Autodesk Inventor part; units mm, degrees
ref_plane "YZ Plane" through (0, 0, 0) normal (1, 0, 0) x (0, 1, 0)
ref_plane "XZ Plane" through (0, 0, 0) normal (0, 1, 0) x (-1, 0, 0)
ref_plane "XY Plane" through (0, 0, 0) normal (0, 0, 1) x (1, 0, 0)
sketch "Sketch1" plane through (0, 0, 0) normal (0, 0, 1) x (1, 0, 0)
  circle A0 centre (0, 0) radius 44.45
  line L0 (-44.45, 44.45) -> (44.45, 44.45)
  line L1 (44.45, 44.45) -> (44.45, -44.45)
  line L2 (44.45, -44.45) -> (-44.45, -44.45)
  line L3 (-44.45, -44.45) -> (-44.45, 44.45)
  dimension "d0" = 88.9
  dimension "d1" = 88.9
  dimension "d2" = 88.9
  dimension "d3" = 44.45
  dimension "d4" = 44.45
extrude "Extrusion1" add sketch "Sketch1" along normal blind 6.35
sketch "Sketch2" plane through (0, 0, 6.35) normal (0, 0, 1) x (1, 0, 0)
  circle A0 centre (0, 0) radius 46.0375
  circle A1 centre (0, 0) radius 44.45
  circle A2 centre (0, 0) radius 39.6875
  dimension "d8" = 1.5875
  dimension "d46" = 88.9
  dimension "d82" = 79.375
extrude "Extrusion2" add sketch "Sketch2" along normal blind 25.4 contours A1
sketch "Sketch3" plane through (0, 0, 6.35) normal (0, 0, 1) x (1, 0, 0)
  circle A0 centre (0, 0) radius 14.2875
  dimension "d11" = 28.575
extrude "Extrusion3" cut sketch "Sketch3" against normal blind 38.1
sketch "Sketch4" plane through (0, 0, 6.35) normal (0, 0, 1) x (1, 0, 0)
  circle A0 centre (0, 0) radius 14.2875
  circle A1 centre (0, 0) radius 19.05
  dimension "d14" = 38.1
extrude "Extrusion4" add sketch "Sketch4" along normal blind 25.4
sketch "Sketch7" plane through (0, 0, 6.35) normal (0, 0, 1) x (1, 0, 0)
  line L0 (44.45, 44.45) -> (0, 44.45)
  line L1 (-44.45, 44.45) -> (-44.45, 0)
  line L2 (-44.45, -44.45) -> (0, -44.45)
  line L3 (44.45, -44.45) -> (44.45, 0)
  line L4 (44.45, -44.45) -> (44.45, 44.45)
  line L5 (-44.45, 0) -> (-44.45, -44.45)
  line L6 (-44.45, -44.45) -> (0, -44.45)
  line L7 (44.45, -44.45) -> (-44.45, -44.45)
  line L8 (0, -44.45) -> (44.45, -44.45)
  line L9 (44.45, -44.45) -> (44.45, 0)
  arc A0 (-44.45, 0) -> (0, -44.45) centre (0, 0) ccw
  arc A1 (0, -44.45) -> (44.45, 0) centre (0, 0) ccw
  arc A2 (44.45, 0) -> (0, 44.45) centre (0, 0) ccw
  line L10 (44.45, 0) -> (44.45, 44.45)
  arc A3 (0, 44.45) -> (-44.45, 0) centre (0, 0) ccw
  line L11 (0, 44.45) -> (-44.45, 44.45)
  arc A4 (-44.45, 0) -> (0, -44.45) centre (0, 0) ccw
  line L12 (-44.45, 0) -> (-44.45, -44.45)
  arc A5 (0, -44.45) -> (44.45, 0) centre (0, 0) ccw
  line L13 (0, -44.45) -> (44.45, -44.45)
  point P0 (-44.4261, -1.4578)
  point P1 (44.4261, -1.4578)
extrude "Extrusion7" [suppressed]
sketch "Sketch8" plane through (0, 0, 0) normal (0, 1, 0) x (-1, 0, 0)
  line L0 (44.45, 6.35) -> (44.45, 31.75)
  arc A0 (44.45, 28.2575) -> (44.45, 22.5425) centre (45.974, 25.4) ccw
  line L1 (44.45, 31.75) -> (-44.45, 31.75)
  line L2 (0, -7.62) -> (0, 45.72)
  arc A1 (44.2147, 22.6811) -> (44.45, 28.2575) centre (45.974, 25.4) ccw
  point P0 (0, 0)
  dimension "d28" = 3.2385
  dimension "d31" = 19.05
  dimension "d45" = 1.7145
revolve "Revolution1" cut sketch "Sketch8" angle 360 about axis through (0, 0, -10) along (0, 0, 1) contours A0 L0
sketch "Sketch11" plane through (0, 0, 0) normal (0, 1, 0) x (-1, 0, 0)
  line L0 (-19.05, 6.35) -> (-19.05, 31.75)
  line L1 (-19.05, 38.1) -> (-26.605, 25.4)
  line L2 (-26.605, 25.4) -> (-23.8011, 25.4)
  line L3 (44.45, 28.2575) -> (-44.45, 28.2575)
  line L4 (-23.8011, 25.4) -> (-17.684, 35.6829)
  point P0 (0, 0)
  dimension "d43" = 25.4
  dimension "d44" = 12.7
sketch "Sketch12" plane through (-44.45, 44.45, 0) normal (0, 1, 0) x (1, 0, 0)
  line L0 (0, 0) -> (88.9, 0)
  line L1 (0, 0) -> (0, -6.35)
  line L2 (44.45, -6.35) -> (0, -6.35)
  line L3 (88.9, 0) -> (88.9, -6.35)
  line L4 (88.9, -6.35) -> (44.45, -6.35)
  point P0 (44.45, 0)
sketch "Sketch13" plane through (0, 0, 0) normal (0, 0, -1) x (-1, 0, 0)
  circle A0 centre (0, 0) radius 44.45
  arc A1 (-44.45, 0) -> (0, -44.45) centre (0, 0) ccw
  line L0 (-7.4513, 43.821) -> (0.0223, 44.45)
  line L1 (0.0223, 44.45) -> (0.2739, 41.4606)
  line L2 (0.2739, 41.4606) -> (-7.1997, 40.8316)
  line L3 (-7.1997, 40.8316) -> (-7.4513, 43.821)
  line L4 (4.1443, 44.2564) -> (11.526, 42.9296)
  line L5 (11.526, 42.9296) -> (10.9953, 39.9769)
  line L6 (10.9953, 39.9769) -> (3.6136, 41.3037)
  line L7 (3.6136, 41.3037) -> (4.1443, 44.2564)
  line L8 (0, 0) -> (0, 70.1731) construction
  line L9 (0, 0) -> (-12.1854, 69.107) construction
  line L10 (0, 0) -> (-24.0006, 65.9411) construction
  line L11 (0, 0) -> (-35.0865, 60.7717) construction
  line L12 (0, 0) -> (-45.1064, 53.7557) construction
  line L13 (0, 0) -> (-53.7557, 45.1064) construction
  line L14 (0, 0) -> (-60.7717, 35.0865) construction
  line L15 (0, 0) -> (-65.9411, 24.0006) construction
  line L16 (0, 0) -> (-69.107, 12.1854) construction
  line L17 (0, 0) -> (-70.1731, 0) construction
  line L18 (0, 0) -> (-69.107, -12.1854) construction
  line L19 (0, 0) -> (-65.9411, -24.0006) construction
  line L20 (0, 0) -> (-60.7717, -35.0865) construction
  line L21 (0, 0) -> (-53.7557, -45.1064) construction
  line L22 (0, 0) -> (-45.1064, -53.7557) construction
  line L23 (0, 0) -> (-35.0865, -60.7717) construction
  line L24 (0, 0) -> (-24.0006, -65.9411) construction
  line L25 (0, 0) -> (-12.1854, -69.107) construction
  line L26 (0, 0) -> (0, -70.1731) construction
  line L27 (0, 0) -> (12.1854, -69.107) construction
  line L28 (0, 0) -> (24.0006, -65.9411) construction
  line L29 (0, 0) -> (35.0865, -60.7717) construction
  line L30 (0, 0) -> (45.1064, -53.7557) construction
  line L31 (0, 0) -> (53.7557, -45.1064) construction
  line L32 (0, 0) -> (60.7717, -35.0865) construction
  line L33 (0, 0) -> (65.9411, -24.0006) construction
  line L34 (0, 0) -> (69.107, -12.1854) construction
  line L35 (0, 0) -> (70.1731, 0) construction
  line L36 (0, 0) -> (69.107, 12.1854) construction
  line L37 (0, 0) -> (65.9411, 24.0006) construction
  line L38 (0, 0) -> (60.7717, 35.0865) construction
  line L39 (0, 0) -> (53.7557, 45.1064) construction
  line L40 (0, 0) -> (45.1064, 53.7557) construction
  line L41 (0, 0) -> (35.0865, 60.7717) construction
  line L42 (0, 0) -> (24.0006, 65.9411) construction
  line L43 (0, 0) -> (12.1854, 69.107) construction
  arc A2 (0, 44.45) -> (-44.45, 0) centre (0, 0) ccw
  line L44 (44.45, 0) -> (43.7747, 7.7187)
  line L45 (43.7747, 7.7187) -> (40.7861, 7.4572)
  line L46 (40.7861, 7.4572) -> (41.4614, -0.2615)
  line L47 (41.4614, -0.2615) -> (44.45, 0)
  circle A3 centre (0, 0) radius 44.45
  line L48 (44.2698, -3.9981) -> (41.3154, -3.4772)
  line L49 (41.3154, -3.4772) -> (40.013, -10.8632)
  line L50 (40.013, -10.8632) -> (42.9675, -11.3842)
  line L51 (44.2698, -3.9981) -> (42.9675, -11.3842)
  dimension "d53" = 7.5
  dimension "d54" = 3
  dimension "d55" = 3
  dimension "d56" = 7.5
  dimension "d59" = 360
  dimension "d61" = 15
  dimension "d95" = 3
  dimension "d98" = 15
  dimension "d99" = 7.5
  dimension "d100" = 3
extrude "Extrusion11" cut sketch "Sketch13" against normal blind 13.35 contours L44 A0 | L47 L46 L45 L44 | L51 L50 L49 L48 | A0 L51
sketch "Sketch14" plane through (0, 0, 0) normal (0, 0, -1) x (-1, 0, 0)
  circle A0 centre (12.472, 29.1978) radius 2.7115
  circle A1 centre (-19.05, 25.4) radius 2.7115
  circle A2 centre (0.2661, -31.7489) radius 2.7115
  circle A3 centre (0, 0) radius 14.2875
  dimension "d64" = 5.4229
  dimension "d71" = 31.75
  dimension "d72" = 31.75
  dimension "d73" = 31.75
  dimension "d74" = 31.75
  dimension "d75" = 60.325
  dimension "d76" = 25.4
extrude "Extrusion12" cut sketch "Sketch14" against normal blind 25.4 contours A0 | A1 | A2
sketch "Sketch15" plane through (0, 0, 0) normal (0, 0, -1) x (-1, 0, 0)
  circle A0 centre (-31.75, 7.75) radius 1.004
  circle A1 centre (-31.75, -7.75) radius 1.004
  circle A2 centre (-31.75, 0) radius 6.35
  point P0 (0, 0)
  dimension "d77" = 7.75
  dimension "d78" = 15.5
  dimension "d79" = 2.008
mirror "Mirror2" about plane through (0, 0, 0) normal (1, 0, 0) of "Extrusion12"
sketch "Sketch16" plane through (0, 0, 6.35) normal (0, 0, 1) x (1, 0, 0)
  circle A0 centre (28.575, 0) radius 5.95
  circle A1 centre (0, 0) radius 14.2875
  dimension "d83" = 11.9
  dimension "d84" = 28.575
extrude "Extrusion14" cut sketch "Sketch16" against normal blind 25.4 contours A0
sketch "Sketch17" plane through (0, 0, 6.35) normal (0, 0, 1) x (1, 0, 0)
  line L0 (23.117, 5.6504) -> (23.117, 7.0495)
  line L1 (25.6612, 6.127) -> (25.6612, -0.8642)
  arc A0 (23.117, 7.0495) -> (25.6612, -0.8642) centre (0.8097, -4.4879) ccw
  arc A1 (25.6612, 6.127) -> (23.117, 5.6504) centre (24.359, 6.0493) ccw
  line L2 (26.9312, -0.7733) -> (26.9312, 5.9401)
  arc A2 (26.9312, 5.9401) -> (21.847, 5.4855) centre (24.359, 6.0493) ccw
  line L3 (21.847, 5.4855) -> (21.847, 11.4358)
  arc A3 (21.847, 11.4358) -> (26.9312, -0.7733) centre (0.8097, -4.4879) ccw
  point P0 (0, 0)
  dimension "d87" = 1.27
extrude "Extrusion15" [suppressed]
sketch "Sketch18" plane through (0, 0, 0) normal (0, 0, -1) x (-1, 0, 0)
  circle A0 centre (-28.575, 19) radius 1
  circle A1 centre (-28.575, -8.3) radius 1
  point P0 (0, 0)
extrude "Extrusion16" cut sketch "Sketch18" against normal blind 25.4
sketch "Sketch19" plane through (0, 0, 0) normal (0, 0, -1) x (-1, 0, 0)
  line L0 (-34.475, 16.6) -> (-22.675, 16.6)
  line L1 (-34.475, 16.6) -> (-34.475, -5.9)
  line L2 (-22.675, -5.9) -> (-22.675, 16.6)
  line L3 (-22.675, -5.9) -> (-34.475, -5.9)
  line L4 (-22.167, 17.108) -> (-34.983, 17.108)
  line L5 (-34.983, 17.108) -> (-34.983, -6.408)
  line L6 (-34.983, -6.408) -> (-22.167, -6.408)
  line L7 (-22.167, -6.408) -> (-22.167, 17.108)
  point P0 (0, 0)
  dimension "d92" = 0.508
extrude "Extrusion17" cut sketch "Sketch19" against normal blind 4.3 contours L0 L2 L3 L1 | L7 L6 L5 L4
sketch "Sketch20" plane through (0, 0, 0) normal (0, 0, -1) x (-1, 0, 0)
  line L0 (0, 44.45) -> (44.45, 44.45)
  line L1 (44.45, 44.45) -> (53.975, 44.45)
  line L2 (53.975, 44.45) -> (53.975, -44.45)
  line L3 (53.975, -44.45) -> (44.45, -44.45)
  line L4 (44.45, -44.45) -> (44.45, 44.45)
  line L5 (-44.45, 44.45) -> (-53.975, 44.45)
  line L6 (-53.975, 44.45) -> (-53.975, -44.45)
  line L7 (-53.975, -44.45) -> (-44.45, -44.45)
  line L8 (-44.45, -44.45) -> (-44.45, 44.45)
  line L9 (-44.45, -44.45) -> (44.45, -44.45)
  line L10 (-44.45, 44.45) -> (-44.45, -44.45)
  point P0 (0, 0)
  dimension "d101" = 9.525
  dimension "d102" = 9.525
extrude "Extrusion18" add sketch "Sketch20" against normal up to surface (6.35 mm away)
sketch "Sketch21" plane through (0, 0, 6.35) normal (0, 0, 1) x (1, 0, 0)
  circle A0 centre (0, 0) radius 44.45
  arc A1 (-43.7747, 7.7187) -> (-44.45, 0) centre (0, 0) ccw
  line L0 (0, -44.45) -> (53.975, -44.45)
  line L1 (53.975, -44.45) -> (43.6252, 8.5234)
  line L2 (-53.975, 44.45) -> (-53.975, -44.45)
  line L3 (-53.975, -44.45) -> (-43.6252, 8.5234)
  line L4 (53.975, 44.45) -> (53.975, -44.45)
  line L5 (53.975, -44.45) -> (53.975, 44.45)
  line L6 (53.975, 44.45) -> (0, 44.45)
  line L7 (-53.975, 44.45) -> (-53.975, -44.45)
  arc A2 (43.6252, 8.5234) -> (0, 44.45) centre (0, 0) ccw
  line L8 (0, 44.45) -> (-53.975, 44.45)
  arc A3 (0, 44.45) -> (-43.6252, 8.5234) centre (0, 0) ccw
extrude "Extrusion19" cut sketch "Sketch21" against normal up to surface (6.35 mm away) contours A0 L6 L4 L1 | A0 L3 L2 L8
fillet "Fillet1" radius 6.35 2 edges at (53.975, -44.45, 3.175) (-53.975, -44.45, 3.175)
equation "\"d55\" = d54"
equation "\"d56\" = d53"
equation "\"d95\" = d54"
equation "\"d99\" = d53"
equation "\"d100\" = d54"
equation "\"d77\" = 0.5 * d78"
equation "\"d102\" = d101"
properties part number "mounting plate" material "ABS Plastic"
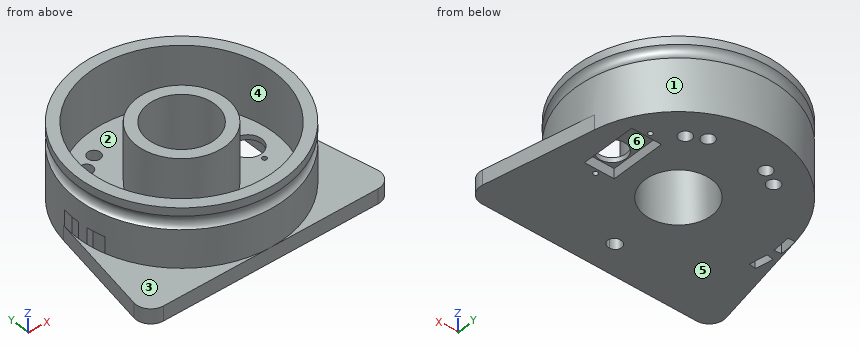
Could you check a few things on this model? Use its own coordinates, in mm. Face numbers are marked on the shaded views. A direction names the side the tool comes from. Round coordinates to 2 decimals unless told otherwise and drop trailing zeros.
(1) I'm going to push flat-ended pins straight in: pin 1 (12 mm diameter, centred on x = -41.5, z = 28, fed in from -Y); pin 2 (10 mm diameter, centred on x = -32, z = 28.5, fed in from -Y); pin 3 (3.5 mm diameter, centred on x = 29, z = 2.5, fed in from +Y). Where does each tip first touch, or does it pass through?
Response values:
pin 1: stops at y = -26.74
pin 2: stops at y = -35.31
pin 3: stops at y = 35.12
(2) Please list where these lines run through material, in increasing order: line 1 along Y through (x, z) = (0, 19); line 2 along Y through (x, z) = (8, 24); line 3 along X through (y, z) = (-6.5, 23).
Response values:
line 1: y = -44.45 to -39.69, -19.05 to -14.29, 14.29 to 19.05, 39.69 to 44.45
line 2: y = -42.3 to -38.87, -17.29 to -11.84, 11.84 to 17.29, 38.87 to 42.3
line 3: x = -43.31 to -39.15, -17.91 to -12.72, 12.72 to 17.91, 39.15 to 43.31
(3) If we mould it in two halves opening along Y, with no side actions, what happens to the marked faces 1, 2 and 3? For each: released by +Y, released by -Y, zero draft, split by the parting line, or undercut.
Response values:
face 1: split by the parting line
face 2: undercut
face 3: zero draft
(4) Imagine slicing it at A-A (z = 16). Count the separate pieces of the cut face and the enclosed holes in it, plus the area to 3 significant figures.
Response values:
separate pieces: 2
enclosed holes: 2
area: 1,760 mm2
(5) Which directions (+Z, -Z, +X, -X, +Y, -Y) give clear straight access to the entire face, cutting with the end or side of a thin tool? Please do the marked faces 4, 5 and 6.
Response values:
face 4: +Z
face 5: -Z, +X, -X, +Y, -Y
face 6: -Z
